```python
from build123d import *

# Parameters (mm, degrees)
F0_R     = 1.15
F1_DEPTH = 1.5


with BuildPart() as f1:
    # F0 (on Front) → F1 (new body)
    with BuildSketch(Plane.XZ):
        with BuildLine():
            Line((-5, 15), (-5, 0))
            Line((-5, 0), (-5, -15))
            Line((-5, -15), (-3.1, -15))
            ThreePointArc((-3.1, -15), (-2.05, -13.95), (-1, -15))
            Line((-1, -15), (-1, -16.8))
            Line((-1, -16.8), (0, -16.8))
            Line((0, -16.8), (1, -16.8))
            Line((1, -16.8), (1, -15))
            ThreePointArc((1, -15), (2.05, -13.95), (3.1, -15))
            Line((3.1, -15), (5, -15))
            Line((5, -15), (5, 0))
            Line((5, 0), (5, 15))
            Line((5, 15), (3.1, 15))
            ThreePointArc((3.1, 15), (2.05, 13.95), (1, 15))
            Line((1, 15), (1, 16.8))
            Line((1, 16.8), (0, 16.8))
            Line((0, 16.8), (-1, 16.8))
            Line((-1, 16.8), (-1, 15))
            ThreePointArc((-1, 15), (-2.05, 13.95), (-3.1, 15))
            Line((-3.1, 15), (-5, 15))
        make_face()
        with Locations((0, -7)):
            Circle(F0_R, mode=Mode.SUBTRACT)
        Circle(F0_R, mode=Mode.SUBTRACT)
        with Locations((0, 7)):
            Circle(F0_R, mode=Mode.SUBTRACT)
    extrude(amount=F1_DEPTH)


solid = f1.part
```
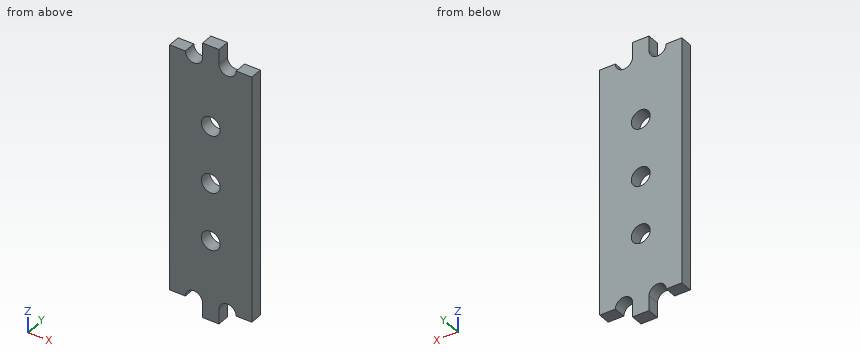
Input: part model. Units: mm. Frame: model coordinates. Give positions to 0.01 mm unless a question says otherwise; leave off trailing zeros. Order: outer loops, then holes, each group sorted by start corner. A loop starts at its lowest first (then second) coordinate and runs counter-clockwise, first axis right, second up. Notation, with made-up numbers: M -29.5,89.25 L -11.5,89.25 A18 ccw -11.5,109.25 Z; hole C 11,88.25 d4. An arc over 180 degrees is marked long. One line per question, with ' | ' between items.
1) Section B-B on x = 0. Output: boundary loops of the cut face in (y, z).
Filled in:
outline: M -1.5,-16.8 L 0,-16.8 L 0,-8.15 L -1.5,-8.15 Z; M -1.5,-5.85 L 0,-5.85 L 0,-1.15 L -1.5,-1.15 Z; M -1.5,1.15 L 0,1.15 L 0,5.85 L -1.5,5.85 Z; M -1.5,8.15 L 0,8.15 L 0,16.8 L -1.5,16.8 Z
2) Section A-A on z = -7. Output: boundary loops of the cut face in (x, y), and give its area (4 significant figures).
Filled in:
outline: M -5,-1.5 L -1.15,-1.5 L -1.15,0 L -5,0 Z; M 1.15,-1.5 L 5,-1.5 L 5,0 L 1.15,0 Z | area: 11.55 mm2
3) Section D-D on x = -3.75. Output: boundary loops of the cut face in (y, z).
Filled in:
outline: M -1.5,-15 L 0,-15 L 0,15 L -1.5,15 Z
4) Section C-C on y = -0.4. Output: boundary loops of the cut face in (x, z), and give its area (3 significant figures).
Filled in:
outline: M -5,-15 L -3.1,-15 A1.05 cw -1,-15 L -1,-16.8 L 1,-16.8 L 1,-15 A1.05 cw 3.1,-15 L 5,-15 L 5,15 L 3.1,15 A1.05 cw 1,15 L 1,16.8 L -1,16.8 L -1,15 A1.05 cw -3.1,15 L -5,15 Z; hole C 0,-7 d2.3; hole C 0,0 d2.3; hole C 0,7 d2.3 | area: 288 mm2
5) Contact query for flat-ended pins moving along their axis: P1, Ø0.8, axis at x = 4, y = -1, coming from the -Z side; P2, Ø3, axis at x = 0, z = 7, coming from the +Y side; P3, Ø0.8, axis at y = -0.5, z = 16.5, coming from the +X side. Output: stop coordinate, or through.
Filled in:
P1: stops at z = -15 | P2: stops at y = 0 | P3: stops at x = 1
6) Ray query, L1, parallel to Z at x = 0, y = -0.85; L2, parallel to Z at x = -3.5, y = -0.6; L3, parallel to X at y = -1.15, z = -7.5. Return the intervals inside material, ascending.
Filled in:
L1: z = -16.8 to -8.15, -5.85 to -1.15, 1.15 to 5.85, 8.15 to 16.8 | L2: z = -15 to 15 | L3: x = -5 to -1.04, 1.04 to 5
